Job drawing, mm, ordinate dimensions from the low corner. One solid piece. A direction names the side the tool comes from. Give positions to 0.01 mm unless a question says otherwise; leave off trailing zeros. Loops run counter-clockwise (first coordinate to the right, second up) from the corner with the lowest first, then second, coordinate; pieces in that order, holes last. Notation, with made-up numbers: M 56,33.25 L 80,33.25 A27 cw 80,66.25 Z; hole C 59.25,53 d4. An arc over 180 degrees is marked long. Answer in a Markdown table with one row per item.
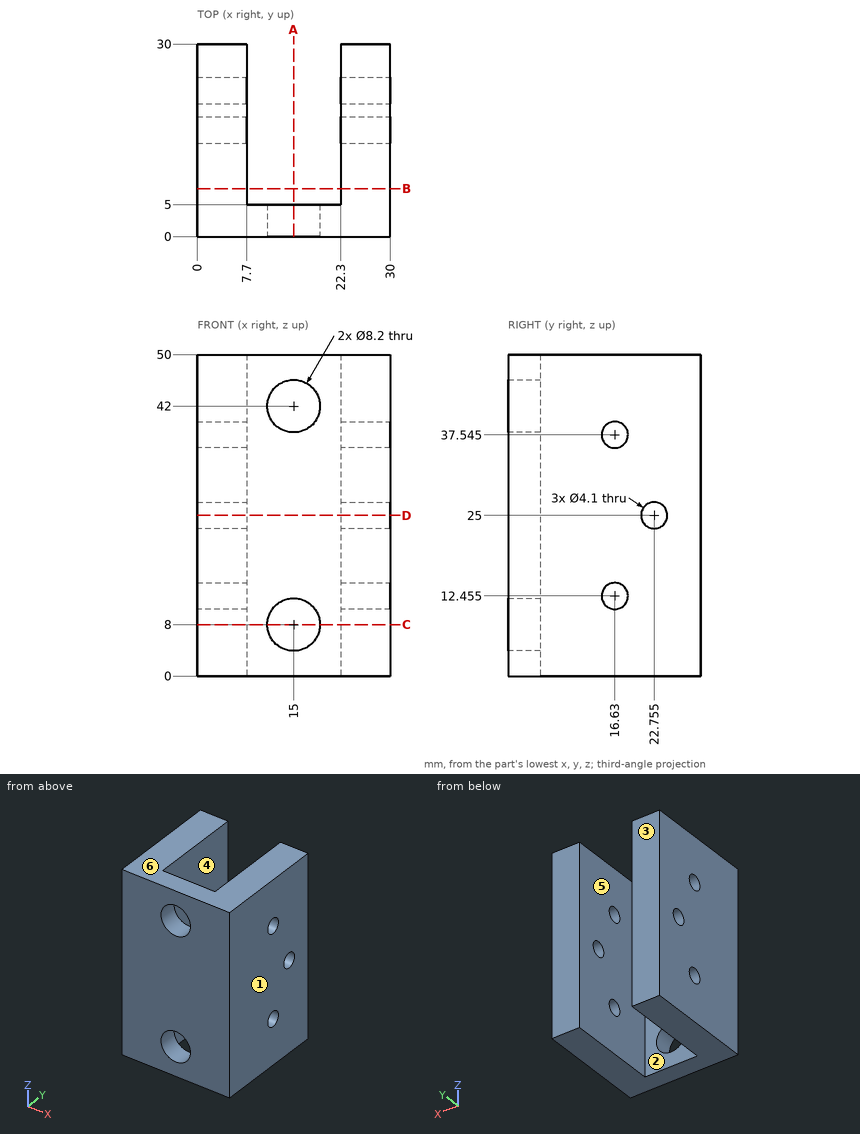
(1) Drill centre lines: line 1 along Z through (x, y) = (25, 15); line 2 along X through (y, z) = (12.75, 15); line 3 along X through (y, z) = (2.1, 42). Where is each one in solid material? Low to high.
Recorded:
| item | result |
|---|---|
| line 1 | z = 0 to 11.21, 13.7 to 36.3, 38.79 to 50 |
| line 2 | x = 0 to 7.7, 22.3 to 30 |
| line 3 | x = 0 to 10.9, 19.1 to 30 |
(2) Saw through at A-A (x = 15). Write the cut outline in (y, z).
Recorded:
| item | result |
|---|---|
| outline | M 0,0 L 5,0 L 5,3.9 L 0,3.9 Z; M 0,12.1 L 5,12.1 L 5,37.9 L 0,37.9 Z; M 0,46.1 L 5,46.1 L 5,50 L 0,50 Z |
(3) Pin check, flat tips, straight feed: pin 1 Ø13 at (x, z) = (15, 8) entering from +Y; pin 2 Ø3.5 at (y, z) = (16.63, 37.55) entering from -X. Stop position of each tip, or through.
Recorded:
| item | result |
|---|---|
| pin 1 | stops at y = 5 |
| pin 2 | passes through |
(4) Saw through at D-D (z = 25). Write the cut outline in (x, y) (1 decimal).
Recorded:
| item | result |
|---|---|
| outline | M 0,0 L 30,0 L 30,20.7 L 22.3,20.7 L 22.3,5 L 7.7,5 L 7.7,20.7 L 0,20.7 Z; M 0,24.8 L 7.7,24.8 L 7.7,30 L 0,30 Z; M 22.3,24.8 L 30,24.8 L 30,30 L 22.3,30 Z |
(5) Which spindle directions (+Z, -Z, +X, -X, +Y, -Y) get a long thin tool onto all of the face, cutting with end or side? Do the marked faces 5 and 6. Say none if no direction does.
Recorded:
| item | result |
|---|---|
| face 5 | +Z, -Z, +Y |
| face 6 | +Z, +X, -X, +Y, -Y |
(6) Saw through at B-B (y = 7.5). Write the cut outline in (x, z), plus the area to 3 significant figures.
Recorded:
| item | result |
|---|---|
| outline | M 0,0 L 7.7,0 L 7.7,50 L 0,50 Z; M 22.3,0 L 30,0 L 30,50 L 22.3,50 Z |
| area | 770 mm^2 |
(7) Saw through at C-C (z = 8). Write the cut outline in (x, y), plus the area to 3 significant figures.
Recorded:
| item | result |
|---|---|
| outline | M 0,0 L 10.9,0 L 10.9,5 L 7.7,5 L 7.7,30 L 0,30 Z; M 19.1,0 L 30,0 L 30,30 L 22.3,30 L 22.3,5 L 19.1,5 Z |
| area | 494 mm^2 |
(8) Pull direction X, two halves, no side cores. Call the marked faces 1, 2, 3 and 4: +X half, -X half, draft (parallel to the pull), parting line (faces both ways), or undercut.
Recorded:
| item | result |
|---|---|
| face 1 | +X half |
| face 2 | undercut |
| face 3 | draft |
| face 4 | undercut |
